The model under review builds one solid part; all positions refer to its coordinate system, in mm. Coordinates: 2 decimals unless noted, no trailing zeros.
```python
from build123d import *

# Parameters (mm, degrees)
F0_W     = 220
F0_H     = 50
F0_R     = 2.1
F1_DEPTH = 2


with BuildPart() as f1:
    # F0 (on Front) → F1 (new body)
    with BuildSketch(Plane.XZ):
        with Locations((109.796509, 24.825824)):
            Rectangle(F0_W, F0_H)
        with BuildLine():
            ThreePointArc((111.896509, 13.085015), (108.311585, 11.600091), (109.796509, 15.185015))
            ThreePointArc((109.796509, 15.185015), (111.281433, 14.56994), (111.896509, 13.085015))
        make_face(mode=Mode.SUBTRACT)
        with Locations((9.796509, 24.825824)):
            Circle(F0_R, mode=Mode.SUBTRACT)
        with BuildLine():
            ThreePointArc((109.796509, 34.985015), (108.311585, 38.56994), (111.896509, 37.085015))
            ThreePointArc((111.896509, 37.085015), (111.281433, 35.600091), (109.796509, 34.985015))
        make_face(mode=Mode.SUBTRACT)
        with Locations((209.796509, 24.825824)):
            Circle(F0_R, mode=Mode.SUBTRACT)
    extrude(amount=F1_DEPTH)


solid = f1.part
```
(1) Wall thickness on probe 1 along X at (y, z) = (-1.2, 24); probe 2 along X at (y, z) = (-1.7, 13.5); probe 3 along X at (y, z) = (-1.3, 26.5): over which ranges is each line inside the solid? List them lowest first.
A:
probe 1: x = -0.2 to 7.87, 11.73 to 207.87, 211.73 to 219.8
probe 2: x = -0.2 to 107.74, 111.86 to 219.8
probe 3: x = -0.2 to 8.53, 11.06 to 208.53, 211.06 to 219.8
(2) For pin 1 Ø2.5 at (x, z) = (109.8, 13.09) entering from +Y; pin 2 Ø5.5 at (x, z) = (9.8, 24.83) entering from -Y, all flat-tipped, find the tip position at first contact; note any pin that passes through.
A:
pin 1: passes through
pin 2: stops at y = -2
(3) Draft analysis for pull direction Z (two halves, no side actions). For faces 1 (the face through (108, -2, 25)), 2 (the face through (9.341, -0.986, 22.776)), state which applies: released by +Z, released by -Z, zero draft, split by the parting line, or undercut.
A:
face 1: zero draft
face 2: undercut
